Autodesk Inventor part; units mm, degrees
ref_plane "YZ Plane" through (0, 0, 0) normal (1, 0, 0) x (0, 1, 0)
ref_plane "XZ Plane" through (0, 0, 0) normal (0, 1, 0) x (-1, 0, 0)
ref_plane "XY Plane" through (0, 0, 0) normal (0, 0, 1) x (1, 0, 0)
sketch "Sketch_1" plane through (0, 0, 0) normal (0, 0, 1) x (1, 0, 0)
  line L0 (10, 0) -> (-0.8, 0)
  line L1 (-0.8, 0) -> (-0.8, 2)
  line L2 (-0.8, 2) -> (-0.2226, 3)
  line L3 (-0.2226, 3) -> (0, 3)
  line L4 (0, 3) -> (0, 1.4467)
  arc A0 (0, 1.4467) -> (0.1, 1.3467) centre (0.1, 1.4467) ccw
  line L5 (0.1, 1.3467) -> (0.9, 1.3467)
  line L6 (0.9, 1.3467) -> (1.4, 1.5)
  line L7 (1.4, 1.5) -> (9.6935, 1.5)
  line L8 (9.6935, 1.5) -> (10, 1.1935)
  line L9 (10, 1.1935) -> (10, 0)
  line L10 (10, 0) -> (-0.8, 0)
revolve "Revolution1" add sketch "Sketch_1" angle 360 about axis through (10, 0, 0) along (1, 0, 0)
thread "Thread1"
sketch "Sketch2" plane through (-0.8, 0, 0) normal (-1, 0, 0) x (0, 0, 1)
  point P0 (0, 0)
hole "Hole1" at (-0.8, 0, 0) direction (1, 0, 0) diameter 1.5 depth 2 tip angle 120
sketch "Sketch_3" plane through (-0.8, 0, 0) normal (1, 0, 0) x (0, 0, -1)
  line L0 (-0.75, -0.433) -> (0, -0.866)
  line L1 (0, -0.866) -> (0.75, -0.433)
  line L2 (0.75, -0.433) -> (0.75, 0.433)
  line L3 (0.75, 0.433) -> (0, 0.866)
  line L4 (0, 0.866) -> (-0.75, 0.433)
  line L5 (-0.75, 0.433) -> (-0.75, -0.433)
extrude "Extrusion1" cut sketch "Sketch_3" along normal blind 2
properties part number "CBSTSR3-10" material "鋼、炭素鋼"
Work out the finished part from the listing and answer in its coordinate system (mm). A direction names the side the tool comes from. Round coordinates to 2 decimals unless told otherwise and drop trailing zeros. Write each loop counter-clockwise with the first axis right and the second up, starting at its lowest first coordinate (ties: lowest second). Pieces come first, ordered by that corner, then holes.
1) A tool of negligible diameter and unlimited length cuts with its end or side. For faces 4 (the flat face through (0, 0, 0.75)), 5 (the cylindrical face through (5.6, -1.5, 0.07)), 6 (the flat face through (-0.8, 0, -1)), from which of +Z, -Z, +X, -X, +Y, -Y can it reach the whole face along a straight path? Write none if from no direction.
2) A cutting plane is placed at A-A (x = 5). Give the vertices of the cut face in (y, z), plus the area to 3 significant figures.
3) The mould has two halves that part along Y. Classify faces 1 (the conical face through (1.558, -0.127, -0.028)), 2 (the flat face through (10, 0, 0)), 3 (the cylindrical face through (0.51, -1.07, -0.82)): pulls with the +Y half, pulls with the -Y half, needs draft (parallel to the pull), parting line crosses it, or undercut.
4) Given pin 1 Ø1.5 at (x, y) = (4.5, 0) entering from -Z; pin 2 Ø0.7 at (x, y) = (0.5, 0) entering from -Z; pin 3 Ø2 at (x, z) = (3.5, -1) entering from +Y, each flat-ended and moving along its own axis, determine where each tip first touches the part or whether it passes through.
5) Straight lines are drawn through the part: line 1 (X direction, y = -0.25, z = 1.6); line 2 (Y direction, x = 4.5, z = -0.4); line 3 (Z direction, x = 6, y = 0). For each, find the intervals that lie inside material, in ascending order.
Completed:
1. face 4: -X
1. face 5: +X
1. face 6: +Z, -Z, -X, +Y, -Y
2. outline: circle Ø3 at (0, 0)
2. area: 7.07 mm2
3. face 1: undercut
3. face 2: needs draft
3. face 3: parting line crosses it
4. pin 1: stops at z = -1.5
4. pin 2: stops at z = -1.35
4. pin 3: stops at y = 1.5
5. line 1: x = -0.8 to 0
5. line 2: y = -1.45 to 1.45
5. line 3: z = -1.5 to 1.5
